from build123d import *

# Parameters (mm, degrees)
F0_R     = 2.25
F1_DEPTH = 4


# Not quite as in the source:
# - a feature names something its author has since deleted; it is built from what else it names


with BuildPart() as f1:
    # F0 (on Front) → F1 (new body)
    with BuildSketch(Plane.XZ):
        with BuildLine():
            Line((-7.0467516529, 14.6327305836), (-29.539125133, 25.4644867683))
            ThreePointArc((-29.539125133, 25.4644867683), (-30.4914278163, 24.3161022725), (-31.3991126327, 23.1321362152))
            Line((-31.3991126327, 23.1321362152), (-15.8339072365, 3.6139860008))
            Line((-15.8339072365, 3.6139860008), (-8.7871555836, 7.0075227419))
            Line((-8.7871555836, 7.0075227419), (-7.0467516529, 14.6327305836))
        make_face()
        with BuildLine():
            Line((-1.4915941641, 38.9714658032), (-7.0467516529, 14.6327305836))
            Line((-7.0467516529, 14.6327305836), (0, 11.2391938425))
            Line((0, 11.2391938425), (7.0467516529, 14.6327305836))
            Line((7.0467516529, 14.6327305836), (1.4915941641, 38.9714658032))
            ThreePointArc((1.4915941641, 38.9714658032), (0, 39), (-1.4915941641, 38.9714658032))
        make_face()
        Polygon((0, 11.2391938425), (-7.0467516529, 14.6327305836), (-8.7871555836, 7.0075227419), (-15.8339072365, 3.6139860008), (-10.9574037875, -2.5009559107), (-12.6978077182, -10.1261637524), (-4.8765034491, -10.1261637524), (0, -16.241105664), (4.8765034491, -10.1261637524), (12.6978077182, -10.1261637524), (10.9574037875, -2.5009559107), (15.8339072365, 3.6139860008), (8.7871555836, 7.0075227419), (7.0467516529, 14.6327305836), align=None)
        with Locations((-9.0692451966, -7.2324817016)):
            Circle(F0_R, mode=Mode.SUBTRACT)
        with Locations((0, -11.6)):
            Circle(F0_R, mode=Mode.SUBTRACT)
        with Locations((9.0692451966, -7.2324817016)):
            Circle(F0_R, mode=Mode.SUBTRACT)
        with Locations((-11.3091637813, 2.5812428339)):
            Circle(F0_R, mode=Mode.SUBTRACT)
        with Locations((-5.0330513738, 10.4512388677)):
            Circle(F0_R, mode=Mode.SUBTRACT)
        Polygon((-9.1977509421, -2.0993266316), (-7.376023565, 5.8821825089), (0, 9.4342882455), (7.376023565, 5.8821825089), (9.1977509421, -2.0993266316), (4.0933842599, -8.5), (-4.0933842599, -8.5), align=None, mode=Mode.SUBTRACT)
        with Locations((11.3091637813, 2.5812428339)):
            Circle(F0_R, mode=Mode.SUBTRACT)
        with Locations((5.0330513738, 10.4512388677)):
            Circle(F0_R, mode=Mode.SUBTRACT)
        with BuildLine():
            Line((29.539125133, 25.4644867683), (7.0467516529, 14.6327305836))
            Line((7.0467516529, 14.6327305836), (8.7871555836, 7.0075227419))
            Line((8.7871555836, 7.0075227419), (15.8339072365, 3.6139860008))
            Line((15.8339072365, 3.6139860008), (31.3991126327, 23.1321362152))
            ThreePointArc((31.3991126327, 23.1321362152), (30.4914278163, 24.3161022725), (29.539125133, 25.4644867683))
        make_face()
        with BuildLine():
            Line((38.3262807167, -7.2177701839), (15.8339072365, 3.6139860008))
            Line((15.8339072365, 3.6139860008), (10.9574037875, -2.5009559107))
            Line((10.9574037875, -2.5009559107), (12.6978077182, -10.1261637524))
            Line((12.6978077182, -10.1261637524), (37.6624588637, -10.1261637524))
            ThreePointArc((37.6624588637, -10.1261637524), (38.0221885751, -8.6783164243), (38.3262807167, -7.2177701839))
        make_face()
        with BuildLine():
            Line((4.8765034491, -10.1261637524), (0, -16.241105664))
            Line((0, -16.241105664), (15.5652053962, -35.7592558784))
            ThreePointArc((15.5652053962, -35.7592558784), (16.9214658256, -35.1377858482), (18.252965207, -34.464898972))
            Line((18.252965207, -34.464898972), (12.6978077182, -10.1261637524))
            Line((12.6978077182, -10.1261637524), (4.8765034491, -10.1261637524))
        make_face()
        with BuildLine():
            Line((-4.8765034491, -10.1261637524), (-12.6978077182, -10.1261637524))
            Line((-12.6978077182, -10.1261637524), (-18.252965207, -34.464898972))
            ThreePointArc((-18.252965207, -34.464898972), (-16.9214658256, -35.1377858482), (-15.5652053962, -35.7592558784))
            Line((-15.5652053962, -35.7592558784), (0, -16.241105664))
            Line((0, -16.241105664), (-4.8765034491, -10.1261637524))
        make_face()
        with BuildLine():
            Line((-10.9574037875, -2.5009559107), (-15.8339072365, 3.6139860008))
            Line((-15.8339072365, 3.6139860008), (-38.3262807167, -7.2177701839))
            ThreePointArc((-38.3262807167, -7.2177701839), (-38.0221885751, -8.6783164243), (-37.6624588637, -10.1261637524))
            Line((-37.6624588637, -10.1261637524), (-12.6978077182, -10.1261637524))
            Line((-12.6978077182, -10.1261637524), (-10.9574037875, -2.5009559107))
        make_face()
        with BuildLine():
            Line((-29.539125133, 25.4644867683), (-35.5784666076, 28.3728803368))
            Line((-35.5784666076, 28.3728803368), (-31.3991126327, 23.1321362152))
            ThreePointArc((-31.3991126327, 23.1321362152), (-30.4914278163, 24.3161022725), (-29.539125133, 25.4644867683))
        make_face()
        with BuildLine():
            Line((1.4915941641, 38.9714658032), (0, 45.5065668312))
            Line((0, 45.5065668312), (-1.4915941641, 38.9714658032))
            ThreePointArc((-1.4915941641, 38.9714658032), (0, 39), (1.4915941641, 38.9714658032))
        make_face()
        with BuildLine():
            Line((-38.3262807167, -7.2177701839), (-44.3656221913, -10.1261637524))
            Line((-44.3656221913, -10.1261637524), (-37.6624588637, -10.1261637524))
            ThreePointArc((-37.6624588637, -10.1261637524), (-38.0221885751, -8.6783164243), (-38.3262807167, -7.2177701839))
        make_face()
        with BuildLine():
            Line((31.3991126327, 23.1321362152), (35.5784666076, 28.3728803368))
            Line((35.5784666076, 28.3728803368), (29.539125133, 25.4644867683))
            ThreePointArc((29.539125133, 25.4644867683), (30.4914278163, 24.3161022725), (31.3991126327, 23.1321362152))
        make_face()
        with BuildLine():
            Line((37.6624588637, -10.1261637524), (44.3656221913, -10.1261637524))
            Line((44.3656221913, -10.1261637524), (38.3262807167, -7.2177701839))
            ThreePointArc((38.3262807167, -7.2177701839), (38.0221885751, -8.6783164243), (37.6624588637, -10.1261637524))
        make_face()
        with BuildLine():
            Line((15.5652053962, -35.7592558784), (19.7445593711, -41))
            Line((19.7445593711, -41), (18.252965207, -34.464898972))
            ThreePointArc((18.252965207, -34.464898972), (16.9214658256, -35.1377858482), (15.5652053962, -35.7592558784))
        make_face()
        with BuildLine():
            Line((-18.252965207, -34.464898972), (-19.7445593711, -41))
            Line((-19.7445593711, -41), (-15.5652053962, -35.7592558784))
            ThreePointArc((-15.5652053962, -35.7592558784), (-16.9214658256, -35.1377858482), (-18.252965207, -34.464898972))
        make_face()
        with BuildLine():
            Line((0, 45.5065668312), (-35.5784666076, 28.3728803368))
            Line((-35.5784666076, 28.3728803368), (-29.539125133, 25.4644867683))
            ThreePointArc((-29.539125133, 25.4644867683), (-16.9214658256, 35.1377858482), (-1.4915941641, 38.9714658032))
            Line((-1.4915941641, 38.9714658032), (0, 45.5065668312))
        make_face()
        with BuildLine():
            Line((-31.3991126327, 23.1321362152), (-35.5784666076, 28.3728803368))
            Line((-35.5784666076, 28.3728803368), (-44.3656221913, -10.1261637524))
            Line((-44.3656221913, -10.1261637524), (-38.3262807167, -7.2177701839))
            ThreePointArc((-38.3262807167, -7.2177701839), (-38.0221885751, 8.6783164243), (-31.3991126327, 23.1321362152))
        make_face()
        with BuildLine():
            Line((35.5784666076, 28.3728803368), (0, 45.5065668312))
            Line((0, 45.5065668312), (1.4915941641, 38.9714658032))
            ThreePointArc((1.4915941641, 38.9714658032), (16.9214658256, 35.1377858482), (29.539125133, 25.4644867683))
            Line((29.539125133, 25.4644867683), (35.5784666076, 28.3728803368))
        make_face()
        with BuildLine():
            Line((44.3656221913, -10.1261637524), (35.5784666076, 28.3728803368))
            Line((35.5784666076, 28.3728803368), (31.3991126327, 23.1321362152))
            ThreePointArc((31.3991126327, 23.1321362152), (37.051082256, 12.1744529102), (39, 0))
            ThreePointArc((39, 0), (38.8312048999, -3.62457253), (38.3262807167, -7.2177701839))
            Line((38.3262807167, -7.2177701839), (44.3656221913, -10.1261637524))
        make_face()
        with BuildLine():
            Line((19.7445593711, -41), (44.3656221913, -10.1261637524))
            Line((44.3656221913, -10.1261637524), (37.6624588637, -10.1261637524))
            ThreePointArc((37.6624588637, -10.1261637524), (30.4914278163, -24.3161022725), (18.252965207, -34.464898972))
            Line((18.252965207, -34.464898972), (19.7445593711, -41))
        make_face()
        with BuildLine():
            Line((-15.5652053962, -35.7592558784), (-19.7445593711, -41))
            Line((-19.7445593711, -41), (19.7445593711, -41))
            Line((19.7445593711, -41), (15.5652053962, -35.7592558784))
            ThreePointArc((15.5652053962, -35.7592558784), (0, -39), (-15.5652053962, -35.7592558784))
        make_face()
        with BuildLine():
            Line((-37.6624588637, -10.1261637524), (-44.3656221913, -10.1261637524))
            Line((-44.3656221913, -10.1261637524), (-19.7445593711, -41))
            Line((-19.7445593711, -41), (-18.252965207, -34.464898972))
            ThreePointArc((-18.252965207, -34.464898972), (-30.4914278163, -24.3161022725), (-37.6624588637, -10.1261637524))
        make_face()
    extrude(amount=F1_DEPTH)


solid = f1.part
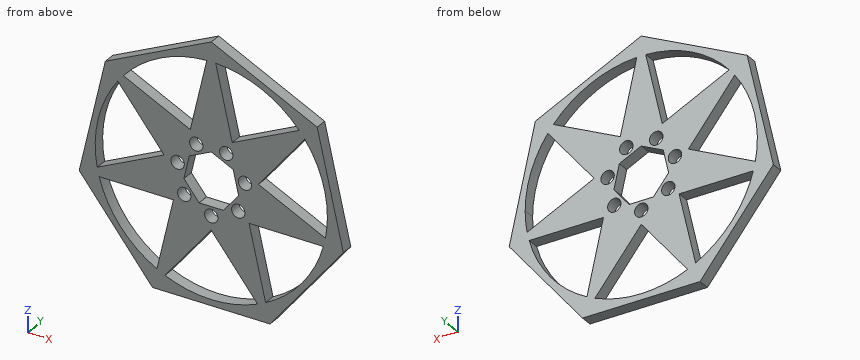
Model file for the job. Use its own axes, mm. Give positions to 0.01 mm unless a question says otherwise; leave off trailing zeros. Loops run counter-clockwise (first coordinate to the right, second up) from the corner with the lowest first, then second, coordinate; pieces in that order, holes last.
1) Wall check: line 1 (X direction, y = -3.5, z = 24.5); line 2 (Z direction, x = -9.5, y = -3.65); line 3 (X direction, y = -2.3, z = 21.5). Give the ranges that are in metal, low to high.
2) Saw through at B-B (z = -11.6). Write the cut outline in (x, y).
3) Flat gauge pin, fed straight in: pin 1 Ø1 at (x, y) = (26.5, -1) entering from +Z. Where does the tip first touch, or does it go through?
4) Saw through at A-A (x = 32.5). Write the cut outline in (y, z).
5) Saw through at C-C (y = -2.1). Count the separate pieces of the cut face and the enclosed holes in it, plus the area to 3 significant figures.
Answer block:
1. line 1: x = -36.46 to -27.54, -4.79 to 4.79, 27.54 to 36.46
1. line 2: z = -41 to -37.83, -28.15 to -9.44, -5.02 to 1.24, 3.92 to 15.81, 37.83 to 40.93
1. line 3: x = -37.15 to -32.54, -30.1 to -21.31, -5.48 to 5.48, 21.31 to 30.1, 32.54 to 37.15
2. outline: (-43.19, -4) - (-37.23, -4) - (-37.23, 0) - (-43.19, 0) - close; (-13.03, -4) - (-2.25, -4) - (-2.25, 0) - (-13.03, 0) - close; (2.25, -4) - (13.03, -4) - (13.03, 0) - (2.25, 0) - close; (37.23, -4) - (43.19, -4) - (43.19, 0) - (37.23, 0) - close
3. pin 1: stops at z = 32.99
4. outline: (-4, -25.01) - (0, -25.01) - (0, -21.56) - (-4, -21.56) - close; (-4, -10.13) - (0, -10.13) - (0, -4.41) - (-4, -4.41) - close; (-4, 21.56) - (0, 21.56) - (0, 29.86) - (-4, 29.86) - close
5. separate pieces: 1
5. enclosed holes: 15
5. area: 2,710 mm2
